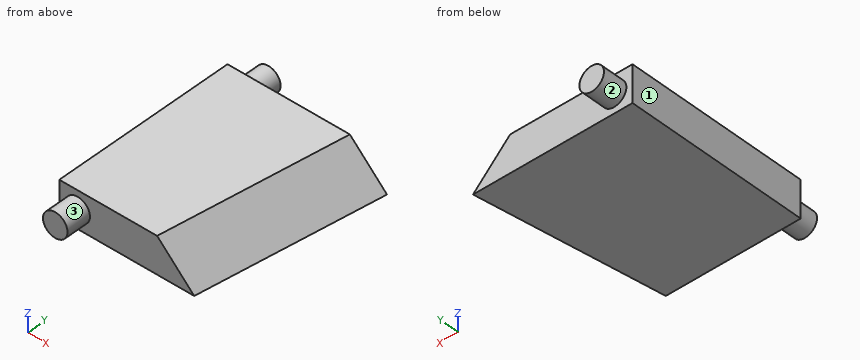
from build123d import *

# Parameters (mm, degrees)
F1_DEPTH = 3
F2_SIZE2 = 2.99999
F2_SIZE  = 2.99999
F3_R     = 1
F4_DEPTH = 2
F5_R     = 1
F6_DEPTH = 2


# Not quite as in the source:
# - a fillet or chamfer is up to 0.001 mm smaller than in the source, because OpenCascade refuses the exact size


with BuildPart() as f1:
    # F0 (on Top) → F1 (new body)
    with BuildSketch(Plane.XY):
        Polygon((11, 3), (11, 0), (22, 0), (24, 15), (11, 15), (11, 12), align=None)
    extrude(amount=F1_DEPTH)

    # F2 (size 3 and 3 in the source; OpenCascade refuses exactly that, so slightly less here)
    f2_edges = [f1.edges().sort_by_distance(p)[0] for p in [
        (23, 7.5, 3),
    ]]
    chamfer(f2_edges, length=F2_SIZE, length2=F2_SIZE2)

    # F3 (on face) → F4 (join)
    with BuildSketch(Plane.XZ):
        with Locations((12.5, 1.5)):
            Circle(F3_R)
    extrude(amount=F4_DEPTH)

    # F5 (on face) → F6 (join)
    with BuildSketch(Plane(origin=(0, 15, 0), x_dir=(-1, 0, 0), z_dir=(0, 1, 0))):
        with Locations((-12.5, 1.5)):
            Circle(F5_R)
    extrude(amount=F6_DEPTH)


solid = f1.part
Verification items for the finished model (mm, model axes). Face numbers are marked on the shaded views. A direction names the side the tool comes from. Give positions to 0.01 mm unless a question says otherwise; leave off trailing zeros. Loops run counter-clockwise (first coordinate to the right, second up) from the corner with the lowest first, then second, coordinate; pieces in that order, holes last. Notation, with made-up numbers: (-6, -25) - (52, -25) arc R26 ccw to (52, 5) - close; hole circle Ø4 at (-18, 83). An arc over 180 degrees is marked (long way). Write item = value, one per line. Start each with the question number.
Q1. Cross-section at C-C, the plane y = -0.5. Enter the section's corners in (x, z), and give its area (3 significant figures).
Q2. Cross-section at A-A, the plane x = 12.5. Enter the section's corners in (y, z).
Q3. Cross-section at B-B, the plane z = 1.85. Enter the section's corners in (x, y).
Q4. Thickness scan on line 1 (Y direction, x = 20, z = 1.6); line 2 (X direction, y = 2.5, z = 1.1); line 3 (X direction, y = 13.75, z = 1.85). Record the ranges inside material, lowest first.
Q5. Depth check by flat-ended pin: P1, Ø0.9, axis at x = 20.5, z = 1.5, coming from the +Y side. Enter the tip coordinate at first touch or a pass-through.
Q6. Tool access check on the marked faces 1, 2 and 3. Record the directions out of +Z, -Z, +X, -X, +Y, -Y that give a thin tool (end or side, any length) a straight path to the whole face; none if there is none.
Answer key:
q1.outline = circle Ø2 at (12.5, 1.5)
q1.area = 3.14 mm^2
q2.outline = (-2, 0.5) - (0, 0.5) - (0, 0) - (15, 0) - (15, 0.5) - (17, 0.5) - (17, 2.5) - (15, 2.5) - (15, 3) - (0, 3) - (0, 2.5) - (-2, 2.5) - close
q3.outline = (11, 0) - (11.56, 0) - (11.56, -2) - (13.44, -2) - (13.44, 0) - (20.13, 0) - (22.13, 15) - (13.44, 15) - (13.44, 17) - (11.56, 17) - (11.56, 15) - (11, 15) - close
q4.line_1 = 0 to 15
q4.line_2 = 11 to 21.22
q4.line_3 = 11 to 21.97
q5.P1 = 15
q6.face_1 = +Z, -Z, -X, +Y, -Y
q6.face_2 = +Y
q6.face_3 = -Y
